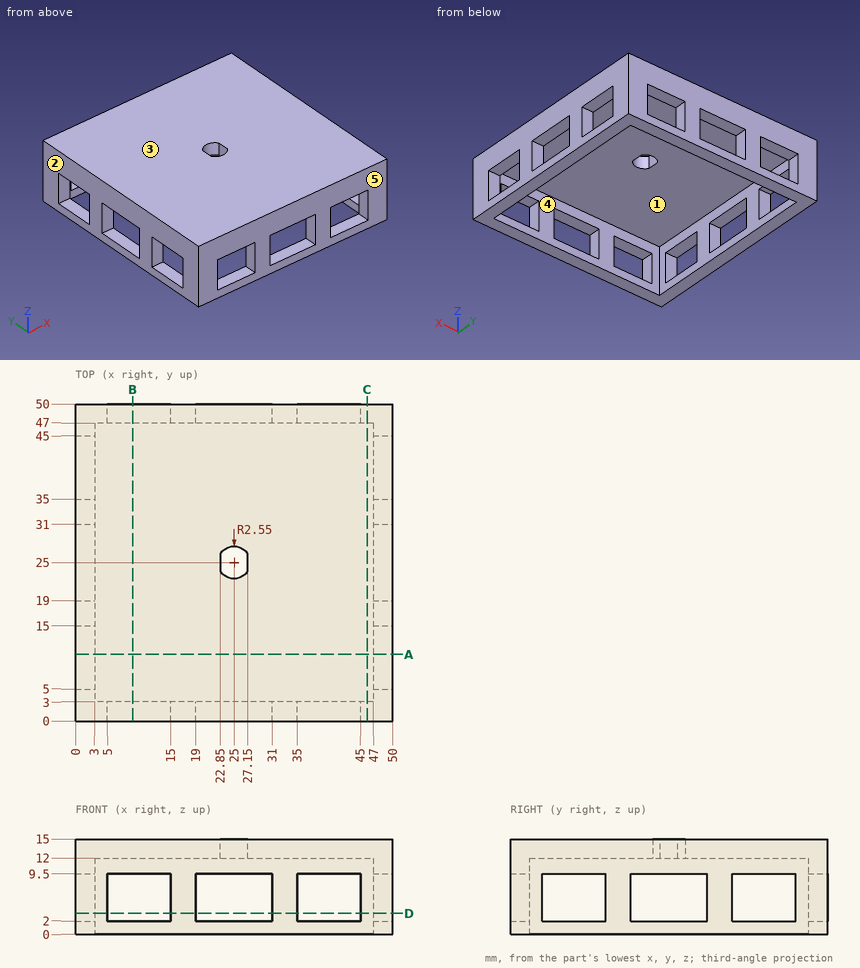
The figure shows three views and two pictorial views of one solid part (mm, origin at its lowest corner). Answer the questions. A direction names the side the tool comes from. Give positions to 0.01 mm unless a question says otherwise; leave off trailing zeros. Loops run counter-clockwise (first coordinate to the right, second up) from the corner with the lowest first, then second, coordinate; pieces in that order, holes last. Notation, with made-up numbers: (29, 33) - (59, 33) arc R25 cw to (59, 58) - close; hole circle Ø5 at (68.25, 62.5). An arc over 180 degrees is marked (long way). Answer in a Markdown table with one row per item.
(1) Section C-C (x = 46) is taken. Give the vertices of the cut face in (y, z).
Results list:
| item | result |
|---|---|
| outline | (0, 0) - (3, 0) - (3, 12) - (47, 12) - (47, 0) - (50, 0) - (50, 15) - (0, 15) - close |
(2) For a pull along X with two mould halves and no side action, classify the marked faces 1, 2 and 3 as pulls with the +X half, pulls with the -X half, needs draft (parallel to the pull), parting line crosses it, or undercut.
Results list:
| item | result |
|---|---|
| face 1 | undercut |
| face 2 | pulls with the -X half |
| face 3 | needs draft |
(3) Section D-D (z = 3.25) is taken. State how many separate pieces and enclosed holes the cut face has, and give its area (3 significant figures).
Results list:
| item | result |
|---|---|
| separate pieces | 12 |
| enclosed holes | 0 |
| area | 180 mm² |
(4) Section A-A (y = 10.5) is taken. Give the vertices of the cut face in (x, z).
Results list:
| item | result |
|---|---|
| outline | (0, 0) - (3, 0) - (3, 2) - (0, 2) - close; (0, 9.5) - (3, 9.5) - (3, 12) - (47, 12) - (47, 9.5) - (50, 9.5) - (50, 15) - (0, 15) - close; (47, 0) - (50, 0) - (50, 2) - (47, 2) - close |
(5) Consider L1, parallel to X at y = 13.5, z = 10.25; L2, parallel to Z at x = 28, y = 48. Determine where each line is inside the solid, lowest interval first. Write a range as [from, to].
Results list:
| item | result |
|---|---|
| L1 | x = [0, 3], [47, 50] |
| L2 | z = [0, 2], [9.5, 15] |
(6) A tool of negligible diameter and unlimited length cuts with its end or side. For the marked faces 4 and 5, from which of +Z, -Z, +X, -X, +Y, -Y can it reach the whole face along a straight path? Write none if from no direction.
Results list:
| item | result |
|---|---|
| face 4 | -Z |
| face 5 | +Z, -Z, +X, -X, -Y |
